The figure shows three views and two pictorial views of one solid part (mm, origin at its lowest corner). Answer the questions. Give positions to 0.01 mm unless a question says otherwise; leave off trailing zeros. Write each loop counter-clockwise with the first axis right and the second up, starting at its lowest first coordinate (ties: lowest second). Pieces come first, ordered by that corner, then holes. Notation, with made-up numbers: (0.25, -30.75) -> (36.25, -30.75) arc R25 cw to (36.25, -3.75) -> close; hole circle Ø6 at (-21.5, 67.5). An arc over 180 degrees is marked (long way). Write item = value, one per line. Start each with the question number.
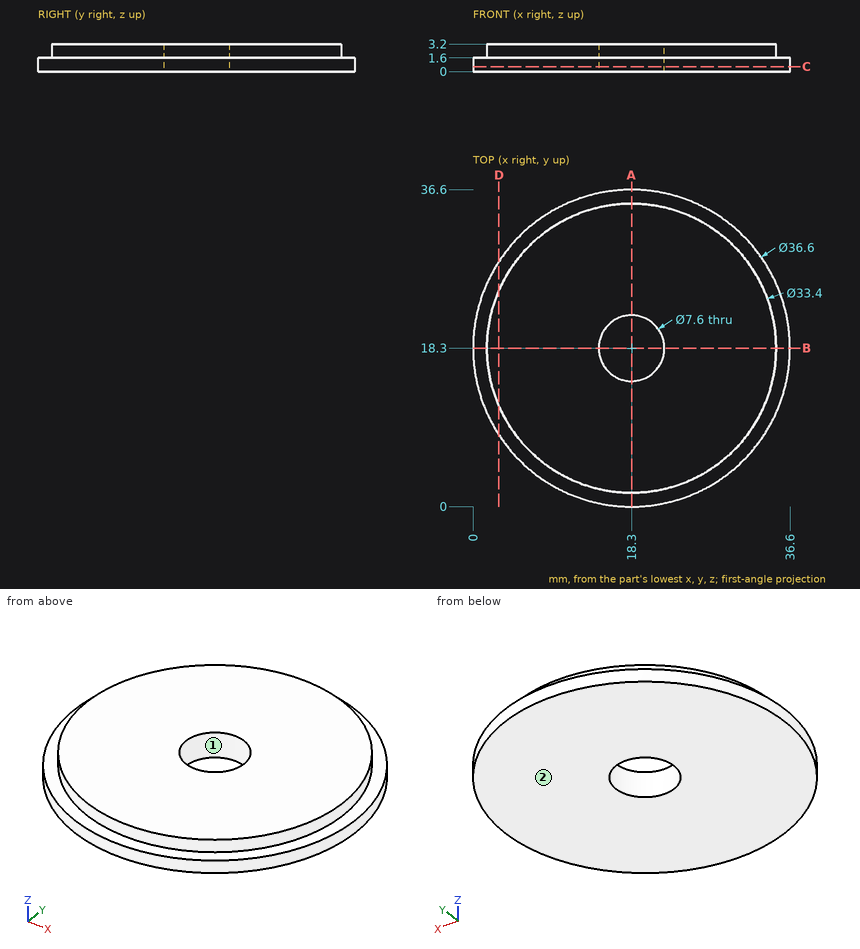
(1) A cutting plane is placed at D-D, the plane x = 3. Write down the section's boundary in (y, z), then the cut area to 3 significant figures.
(2) Find the intervals of material crossed by line 1 along Y through (x, z) = (18.3, 2.25); line 2 along Y through (x, z) = (18.3, 0.95); line 3 along Z through (x, y) = (22.5, 2), in increasing order.
(3) A cutting plane is placed at A-A, the plane x = 18.3. Write down the section's boundary in (y, z), then the cut area to 3 significant figures.
(4) Determine the mould class of the marked faces 1 and 2 for opening direction X: pulls with the +X half, pulls with the -X half, needs draft (parallel to the pull), parting line crosses it, or undercut.
(5) Each of these flat-tipped pins is pushed along its axis until it touches: pin 1 (1 mm diameter, centred on x = 26, z = 2.5, fed in from -Y); pin 2 (1.5 mm diameter, centred on x = 7, z = 2, fed in from -Y); pin 3 (1 mm diameter, centred on x = 4, z = 1.5, fed in from +Y). Where does it stop, or does it pass through?
(6) A cutting plane is placed at C-C, the plane z = 0.6. Write down the section's boundary in (x, y).
Results list:
q1.outline = (8.26, 0) -> (28.34, 0) -> (28.34, 1.6) -> (24.99, 1.6) -> (24.99, 3.2) -> (11.61, 3.2) -> (11.61, 1.6) -> (8.26, 1.6) -> close
q1.area = 53.5 mm²
q2.line_1 = 1.6 to 14.5, 22.1 to 35
q2.line_2 = 0 to 14.5, 22.1 to 36.6
q2.line_3 = 0 to 1.6
q3.outline = (0, 0) -> (14.5, 0) -> (14.5, 3.2) -> (1.6, 3.2) -> (1.6, 1.6) -> (0, 1.6) -> close; (22.1, 0) -> (36.6, 0) -> (36.6, 1.6) -> (35, 1.6) -> (35, 3.2) -> (22.1, 3.2) -> close
q3.area = 87.7 mm²
q4.face_1 = undercut
q4.face_2 = needs draft
q5.pin_1 = 3.23
q5.pin_2 = 3.43
q5.pin_3 = 30.32
q6.outline = circle Ø36.6 at (18.3, 18.3); hole circle Ø7.6 at (18.3, 18.3)
